from build123d import *

# Parameters (mm, degrees)
ESQUISSE1_W                = 58
ESQUISSE1_H                = 18
BOSS_EXTRU_1_DEPTH         = 5
R_P_TITION_LIN_AIRE1_COUNT = 2
R_P_TITION_LIN_AIRE1_PITCH = 40


with BuildPart() as part:
    # Esquisse1 → Boss.-Extru.1 (new body)
    with BuildSketch(Plane.XY):
        Rectangle(ESQUISSE1_W, ESQUISSE1_H)
    extrude(amount=BOSS_EXTRU_1_DEPTH)

    # Esquisse3 → Fraisage pour vis à tête fraisée à 6 pans creux M61 (revolve, cut)
    with BuildSketch(Plane(origin=(20, 0, 5), x_dir=(0, -1, 0), z_dir=(1, 0, 0))):
        Polygon((0, 0), (0, 5), (3.25, 5), (3.25, 4), (7.25, 0), align=None)
    fraisage_pour_vis_t_te_frais_e_6_pan = revolve(axis=Axis((20, 0, 11.35), (0, 0, -1)), mode=Mode.SUBTRACT)

    # Répétition linéaire1: Fraisage pour vis à tête fraisée à 6 pans creux M61 ×2
    with Locations(*[(-i * R_P_TITION_LIN_AIRE1_PITCH, 0, 0) for i in range(1, R_P_TITION_LIN_AIRE1_COUNT)]):
        add(fraisage_pour_vis_t_te_frais_e_6_pan, mode=Mode.SUBTRACT)


solid = part.part
Input: part model. Units: mm. Frame: model coordinates. Coordinates: 2 decimals unless noted, no trailing zeros. Loops run counter-clockwise (first coordinate to the right, second up) from the corner with the lowest first, then second, coordinate; pieces in that order, holes last. Notation, with made-up numbers: (-35.5, 20.5) - (-29.5, 20.5) arc R29 cw to (-29.5, 47.5) - close; hole circle Ø7 at (-35.75, 23). An arc over 180 degrees is marked (long way). Answer in a Markdown table with one row per item. Add a question column.
Item 1: Section query C-C on x = 20. Return the cut outline in (y, z).
Item 2: Line query: line 1 along X through (y, z) = (0, 0.5); line 2 along Y through (x, z) = (-20, 0.4); line 3 along X through (y, z) = (1, 4.35). Output: solid intervals per line, ascending. Write a range as [from, to].
Item 3: Section query B-B on z = 4.35. Return the cut outline in (x, y), then the cut area to 3 significant figures.
Item 4: Contact query for flat-ended pins moving along their axis: P1, Ø8.5, axis at x = 20, y = 0, coming from the +Z side; P2, Ø2, axis at x = 4.5, y = 6, coming from the -Z side. Output: stop coordinate, or through.
Item 5: Section query D-D on z = 0.5. Return the cut outline in (x, y), then the cut area to 3 significant figures.
Item 6: Mould query, pull axis X, two halves, no side actions, for faces 1 (the flat face through (0, 0, 5)), 2 (the cylindrical face through (-16.827, 0.705, 0.507)), 3 (the flat face through (29, 0, 2)), 4 (the cylindrical face through (16.778, 0.423, 0.507)). Classes: released by +X, released by -X, zero draft, split by the parting line, or undercut.
Item 7: Section query A-A on y = 0. Return the cut outline in (x, z), then the cut area to 3 significant figures.
Recorded:
| question | item | result |
|---|---|---|
| 1 | outline | (-9, 0) - (-3.25, 0) - (-3.25, 1) - (-7.25, 5) - (-9, 5) - close; (3.25, 0) - (9, 0) - (9, 5) - (7.25, 5) - (3.25, 1) - close |
| 2 | line 1 | [-29, -23.25], [-16.75, 16.75], [23.25, 29] |
| 2 | line 2 | [-9, -3.25], [3.25, 9] |
| 2 | line 3 | [-29, -26.52], [-13.48, 13.48], [26.52, 29] |
| 3 | outline | (-29, -9) - (29, -9) - (29, 9) - (-29, 9) - close; hole circle Ø13.2 at (-20, 0); hole circle Ø13.2 at (20, 0) |
| 3 | area | 770 mm^2 |
| 4 | P1 | z = 2 |
| 4 | P2 | z = 0 |
| 5 | outline | (-29, -9) - (29, -9) - (29, 9) - (-29, 9) - close; hole circle Ø6.5 at (-20, 0); hole circle Ø6.5 at (20, 0) |
| 5 | area | 978 mm^2 |
| 6 | face 1 | zero draft |
| 6 | face 2 | undercut |
| 6 | face 3 | released by +X |
| 6 | face 4 | undercut |
| 7 | outline | (-29, 0) - (-23.25, 0) - (-23.25, 1) - (-27.25, 5) - (-29, 5) - close; (-16.75, 0) - (16.75, 0) - (16.75, 1) - (12.75, 5) - (-12.75, 5) - (-16.75, 1) - close; (23.25, 0) - (29, 0) - (29, 5) - (27.25, 5) - (23.25, 1) - close |
| 7 | area | 193 mm^2 |
